Autodesk Inventor part; units mm, degrees
ref_plane "YZ Plane" through (0, 0, 0) normal (1, 0, 0) x (0, 1, 0)
ref_plane "XZ Plane" through (0, 0, 0) normal (0, 1, 0) x (-1, 0, 0)
ref_plane "XY Plane" through (0, 0, 0) normal (0, 0, 1) x (1, 0, 0)
sketch "Sketch1" plane through (0, 0, 0) normal (0, 1, 0) x (-1, 0, 0)
  arc A0 (5.4, 2.6153) -> (5.4, -2.6153) centre (0, 0) ccw
  line L0 (1.65, 1.65) -> (-1.65, 1.65)
  line L1 (-1.65, 1.65) -> (-1.65, -1.65)
  line L2 (-1.65, -1.65) -> (1.65, -1.65)
  line L3 (1.65, -1.65) -> (1.65, 1.65)
  line L4 (1.65, 1.65) -> (-1.65, -1.65) construction
  line L5 (-1.65, 1.65) -> (1.65, -1.65) construction
  line L6 (5.4, -2.6153) -> (5.4, 2.6153)
  circle A1 centre (2.5, 2.5) radius 1.1
  circle A2 centre (2.5, -2.5) radius 1.1
  circle A3 centre (-2.5, 2.5) radius 1.1
  circle A4 centre (-2.5, -2.5) radius 1.1
  point P0 (-6, 0)
  dimension "d0" = 12
  dimension "d1" = 3.3
  dimension "d2" = 3.3
  dimension "d3" = 11.4
  dimension "d4" = 2.2
  dimension "d7" = 5
  dimension "d10" = 5
extrude "Extrusion1" add sketch "Sketch1" along normal blind 5.8 contours L6 A0 | A1 | A2 | A3 | A4
extrude "Extrusion2" add sketch "Sketch1" along normal blind 10.8 contours L3 L2 L1 L0
extrude "Extrusion3" add sketch "Sketch1" against normal blind 5 contours A1 | A2 | A3 | A4
fillet "Fillet1" radius 0.2 4 edges at (0, 10.8, -1.65) (-1.65, 10.8, 0) (0, 10.8, 1.65) (1.65, 10.8, 0)
properties part number "D6L90 F1 LFS"
Read the model definition and answer for the solid it produces. Units are mm, in the model's axes. A direction names the side the tool comes from. Round coordinates to 2 decimals unless told otherwise and drop trailing zeros. Order: outer loops, then holes, each group sorted by start corner. A loop starts at its lowest first (then second) coordinate and runs counter-clockwise, first axis right, second up. Notation, with made-up numbers: (-17.75, 47.5) - (31.25, 47.5) arc R19 ccw to (31.25, 70.5) - close; hole circle Ø2 at (41, 30). An arc over 180 degrees is marked (long way). Use one line per item in the form item = value. Start each with the question number.
(1) The part is cut by section D-D (y = -0.25). Give the vertices of the cut face in (x, z), then the cut area to 3 significant figures.
(2) Find the intervals of material crossed by line 1 along Y through (x, z) = (3.5, 4); line 2 along X through (y, z) = (7, -1.5); line 3 along Z through (x, y) = (-2.75, -1.25), in increasing order. Write a range as from..to.
(3) Determine the mould class of faces 6 (the face through (0, 8, -1.65)), 7 (the face through (-3.55, -2.46, -2.17)), 8 (the face through (-5.4, 3, 0)) for opening direction X: +X half, -X half, draft (parallel to the pull), parting line (faces both ways), or undercut.
(4) The part is cut by section C-C (y = 4.5). Give the vertices of the cut face in (x, z), then the cut area to 3 significant figures.
(5) The part is cut by section B-B (x = 0). Give the vertices of the cut face in (y, z).
(6) For faces 1 (the face through (0, 8, 1.65)), 2 (the face through (-1.65, 8, 0)), 3 (the face through (1.45, -2.46, 2.83)), 4 (the face through (1.65, 8, 0)), 5 (the face through (3, -5, 3)), determine the directions among +Z, -Z, +X, -X, +Y, -Y from which every point of the face is accessible in a straight line to the end or side of a thin tool.
(7) The part is cut by section A-A (z = 0). Give the vertices of the cut face in (x, y), then the cut area to 3 significant figures.
(8) Flat-ended cylindrical pins translate along their axes: pin 1 Ø1 at (x, y) = (0.5, 7) entering from -Z; pin 2 Ø2.5 at (y, z) = (9, 0) entering from +X; pin 3 Ø1.6 at (x, y) = (-0.5, 7.5) entering from +Z. Find the tip coordinate at first contact, or state that the pin passes through.
Checked values:
q1.outline = circle Ø2.2 at (-2.5, -2.5); circle Ø2.2 at (-2.5, 2.5); circle Ø2.2 at (2.5, -2.5); circle Ø2.2 at (2.5, 2.5)
q1.area = 15.2 mm^2
q2.line_1 = 0..5.8
q2.line_2 = -1.65..1.65
q2.line_3 = -3.57..-1.43, 1.43..3.57
q3.face_6 = draft
q3.face_7 = undercut
q3.face_8 = -X half
q4.outline = (-5.4, -2.62) arc R6 ccw (long way) to (-5.4, 2.62) - close
q4.area = 111 mm^2
q5.outline = (0, -6) - (5.8, -6) - (5.8, -1.65) - (10.6, -1.65) arc R0.2 ccw to (10.8, -1.45) - (10.8, 1.45) arc R0.2 ccw to (10.6, 1.65) - (5.8, 1.65) - (5.8, 6) - (0, 6) - close
q6.face_1 = +Z, +X, -X, +Y
q6.face_2 = +Z, -Z, -X, +Y
q6.face_3 = -Y
q6.face_4 = +Z, -Z, +X, +Y
q6.face_5 = +Z, -Z, +X, -X, -Y
q7.outline = (-5.4, 0) - (6, 0) - (6, 5.8) - (1.65, 5.8) - (1.65, 10.6) arc R0.2 ccw to (1.45, 10.8) - (-1.45, 10.8) arc R0.2 ccw to (-1.65, 10.6) - (-1.65, 5.8) - (-5.4, 5.8) - close
q7.area = 82.6 mm^2
q8.pin_1 = -1.65
q8.pin_2 = 1.65
q8.pin_3 = 1.65
